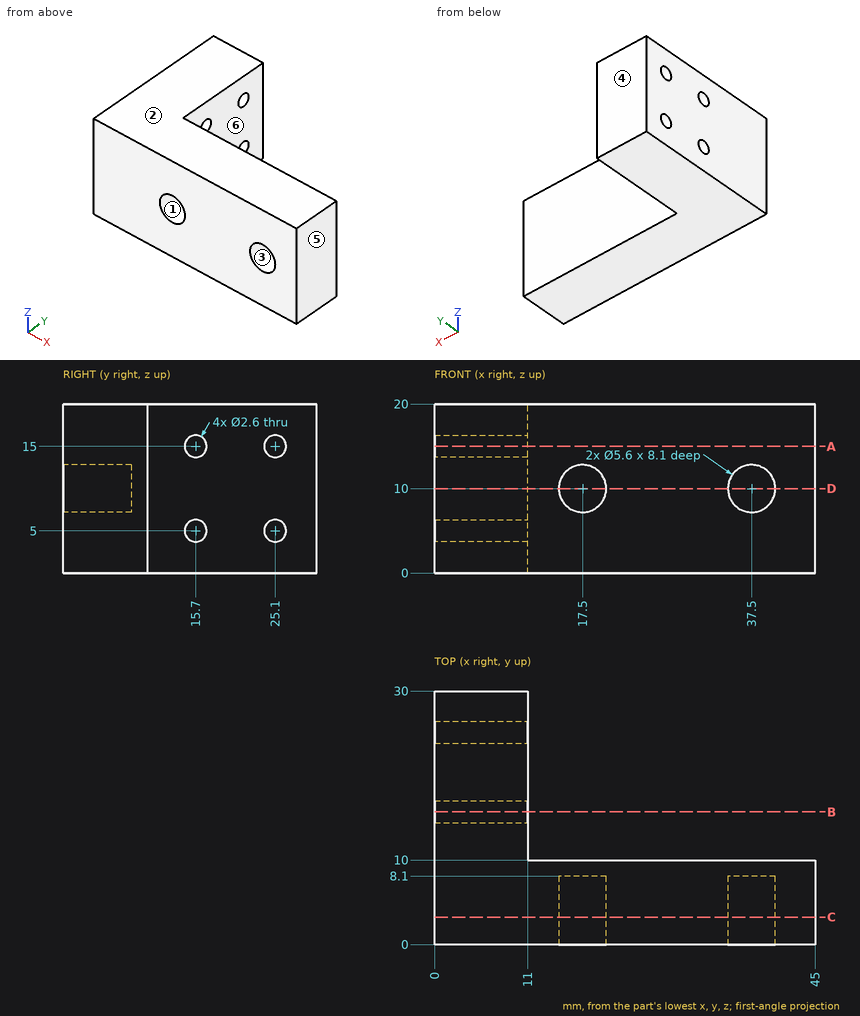
Print and shaded views of the part. All mm, measured from the part's lowest x, y and z. A direction names the side the tool comes from. Round coordinates to 2 decimals unless told otherwise and drop trailing zeros. Write each loop counter-clockwise with the first axis right and the second up, starting at its lowest first coordinate (ties: lowest second). Pieces come first, ordered by that corner, then holes. Notation, with made-up numbers: (38, 85.25) - (76, 85.25) arc R32 ccw to (76, 115.25) - close; hole circle Ø11 at (55.5, -20). An arc over 180 degrees is marked (long way). Write each question's results on one line, items separated by ' | '. Start each with the question number.
Item 1: Wall check: L1, parallel to Y at x = 7, z = 5; L2, parallel to Y at x = 28, z = 6; L3, parallel to X at y = 12.75, z = 5.25. Give the ranges that are in metal, low to high. Write a range as [from, to].
Item 2: Saw through at B-B (y = 15.7). Write the cut outline in (x, z).
Item 3: Drop flat-ended pins along their axis: P1, Ø10, axis at y = 24.5, z = 2, coming from the +X side; P2, Ø1.7, axis at x = 18.5, z = 11.5, coming from the -Y side; P3, Ø3.5, axis at x = 37.5, z = 10, coming from the +Y side. Give the stop position or say it passes through.
Item 4: Saw through at D-D (z = 10). Write the cut outline in (x, y), and give its area (3 significant figures).
Item 5: Mould opens along Z. For the marked faces 1, 2, 3 and 4 say: pulls with the +Z half, pulls with the -Z half, needs draft (parallel to the pull), parting line crosses it, or undercut.
Item 6: Saw through at C-C (y = 3.25). Write the cut outline in (x, z), and give its area (3 significant figures).
Item 7: Saw through at A-A (z = 15). Write the cut outline in (x, y).
Item 8: Which spindle directions (+Z, -Z, +X, -X, +Y, -Y) get a long thin tool onto all of the face, cutting with end or side? Do the marked faces 5 and 6. Say none if no direction does.
Results are:
1) L1: y = [0, 14.4], [17, 23.8], [26.4, 30] | L2: y = [0, 10] | L3: x = [0, 11]
2) outline: (0, 0) - (11, 0) - (11, 3.7) - (0, 3.7) - close; (0, 6.3) - (11, 6.3) - (11, 13.7) - (0, 13.7) - close; (0, 16.3) - (11, 16.3) - (11, 20) - (0, 20) - close
3) P1: stops at x = 11 | P2: stops at y = 8.1 | P3: stops at y = 10
4) outline: (0, 0) - (14.7, 0) - (14.7, 8.1) - (20.3, 8.1) - (20.3, 0) - (34.7, 0) - (34.7, 8.1) - (40.3, 8.1) - (40.3, 0) - (45, 0) - (45, 10) - (11, 10) - (11, 30) - (0, 30) - close | area: 579 mm²
5) face 1: undercut | face 2: pulls with the +Z half | face 3: undercut | face 4: needs draft
6) outline: (0, 0) - (45, 0) - (45, 20) - (0, 20) - close; hole circle Ø5.6 at (17.5, 10); hole circle Ø5.6 at (37.5, 10) | area: 851 mm²
7) outline: (0, 0) - (45, 0) - (45, 10) - (11, 10) - (11, 14.4) - (0, 14.4) - close; (0, 17) - (11, 17) - (11, 23.8) - (0, 23.8) - close; (0, 26.4) - (11, 26.4) - (11, 30) - (0, 30) - close
8) face 5: +Z, -Z, +X, +Y, -Y | face 6: +Z, -Z, +X, +Y
